Autodesk Fusion 360 part; units mm, degrees
sketch "Sketch1" plane through (0, 0, 0) normal (0, 0, 1) x (1, 0, 0)
  line L0 (8.75, 37.75) -> (-8.75, 37.75)
  line L1 (-8.75, 37.75) -> (-8.75, -37.75)
  line L2 (-8.75, -37.75) -> (8.75, -37.75)
  line L3 (8.75, -37.75) -> (8.75, 37.75)
  line L4 (8.75, 37.75) -> (-8.75, -37.75) construction
  line L5 (-8.75, 37.75) -> (8.75, -37.75) construction
  dimension "d1" = 17.5
  dimension "d2" = 75.5
extrude "Extrude1" add sketch "Sketch1" along normal blind 30
fillet "Fillet1" radius 2.5 4 edges at (8.75, 0, 30) (-8.75, 0, 30) (8.75, 0, 0) (-8.75, 0, 0)
sketch "Sketch2" plane through (0, -37.75, 0) normal (0, -1, 0) x (1, 0, 0)
  arc A0 (-8.75, 2.5) -> (-6.25, 0) centre (-6.25, 2.5) ccw
  line L0 (-6.25, 0) -> (6.25, 0)
  arc A1 (6.25, 0) -> (8.75, 2.5) centre (6.25, 2.5) ccw
  line L1 (8.75, 2.5) -> (8.75, 27.5)
  arc A2 (8.75, 27.5) -> (6.25, 30) centre (6.25, 27.5) ccw
  line L2 (6.25, 30) -> (-6.25, 30)
  arc A3 (-6.25, 30) -> (-8.75, 27.5) centre (-6.25, 27.5) ccw
  line L3 (-8.75, 27.5) -> (-8.75, 2.5)
  line L4 (-5.5, 3) -> (5.5, 3)
  line L5 (5.5, 3) -> (5.5, 0)
  line L6 (5.5, 0) -> (-5.5, 0)
  line L7 (-5.5, 0) -> (-5.5, 3)
  dimension "d7" = 11
  dimension "d8" = 3
extrude "Extrude2" add sketch "Sketch2" along normal blind 12 contours L0 L4 L5 L6 L7
Model file for the job. Use its own axes, mm. A direction names the side the tool comes from. Give positions to 0.01 mm unless a question says otherwise; leave off trailing zeros. Order: outer loops, then holes, each group sorted by start corner. A loop starts at its lowest first (then second) coordinate and runs counter-clockwise, first axis right, second up. Notation, with made-up numbers: M 48.25,22.25 L 62.25,22.25 A23 ccw 62.25,30.25 Z; hole C -1,65 d7. An arc over 180 degrees is marked long. Write item = value, one per line.
Q1. Tool access for faces 1 (the flat face through (5.5, -44, 2)), 2 (the cylindrical face through (-7.998, -0.529, 29.287)), 3 (the flat face through (0, -44, 3)), 4 (the flat face through (8.75, -1, 15)), 5 (the flat face through (-5.5, -44, 1)): list every direction of +Z, -Z, +X, -X, +Y, -Y with a clear straight run to the whole face (end or side of a thin tool).
Derived:
face_1 = +Z, -Z, +X, -Y
face_2 = +Z, -X, +Y, -Y
face_3 = +Z, +X, -X, -Y
face_4 = +Z, -Z, +X, +Y, -Y
face_5 = +Z, -Z, -X, -Y
Q2. Cut at B-B, the plane y = -40. List the corners of the cut face in (x, z).
Derived:
outline = M -5.5,0 L 5.5,0 L 5.5,3 L -5.5,3 Z
Q3. Drill centre lines: line 1 (Z direction, x = -6.5, y = -27.5); line 2 (Y direction, x = 2.75, z = 18.75); line 3 (X direction, y = 12, z = 2). Where is each one in solid material? Low to high. Write a range as [from, to].
Derived:
line_1 = [0.01, 29.99]
line_2 = [-37.75, 37.75]
line_3 = [-8.7, 8.7]
Q4. Flat gauge pins, fed straight in: pin 1 (9 mm diameter, centred on x = -1.5, z = 13, fed in from -Y); pin 2 (0.9 mm diameter, centred on y = -44, z = 2, fed in from +X); pin 3 (2.5 mm diameter, centred on y = -41, z = 1, fed in from -X). Where does each tip first touch, or does it go through?
Derived:
pin_1 = -37.75
pin_2 = 5.5
pin_3 = -5.5
Q5. Cut at C-C, the plane z = 7.5. List the corners of the cut face in (x, y), then the cut area to 3 significant figures.
Derived:
outline = M -8.75,-37.75 L 8.75,-37.75 L 8.75,37.75 L -8.75,37.75 Z
area = 1,320 mm2
Q6. Cut at A-A, the plane x = 1.75. List the corners of the cut face in (y, z), then the cut area to 3 significant figures.
Derived:
outline = M -49.75,0 L 37.75,0 L 37.75,30 L -37.75,30 L -37.75,3 L -49.75,3 Z
area = 2,300 mm2
